Could you check a few things on this drawing? It's one solid part, dimensions in mm from its lowest x, y, z. Coordinates: 2 decimals unless noted, no trailing zeros. Loops run counter-clockwise (first coordinate to the right, second up) from the corner with the lowest first, then second, coordinate; pieces in that order, holes last. Notation, with made-up numbers: M 41.25,60.25 L 66.25,60.25 A21 cw 66.25,81.25 Z; hole C 76,86.25 d5. An arc over 180 degrees is marked long. Use one line per item in the form item = value. Start each with the question number.
(1) Please list where these lines run through material, in increasing order: L1, parallel to X at y = 51.64, z = 0.65; L2, parallel to Y at x = 1.75, z = 1.5; L3, parallel to Y at x = 10.25, z = 0.55.
(2) Imagine slicing it at B-B, the plane x = 8.5. Please give me the cut outline in (y, z) (3 decimals).
(3) Imagine slicing it at D-D, the plane x = 13.45. State how many separate pieces and enclosed holes the cut face has, and give its area (3 significant figures).
(4) Imagine slicing it at A-A, the plane y = 10. Please give me the cut outline in (x, z).
(5) Will these pins go through, and if not, where does the flat tip stop? P1, Ø1, axis at x = 7.5, z = 1, coming from the -Y side; P2, Ø0.6, axis at y = 77, z = 0.5, coming from the +X side; P3, Ø1, axis at y = 3.5, z = 1, coming from the -X side.
(6) Imagine slicing it at C-C, the plane y = 31.64. Please give me the cut outline in (x, z).
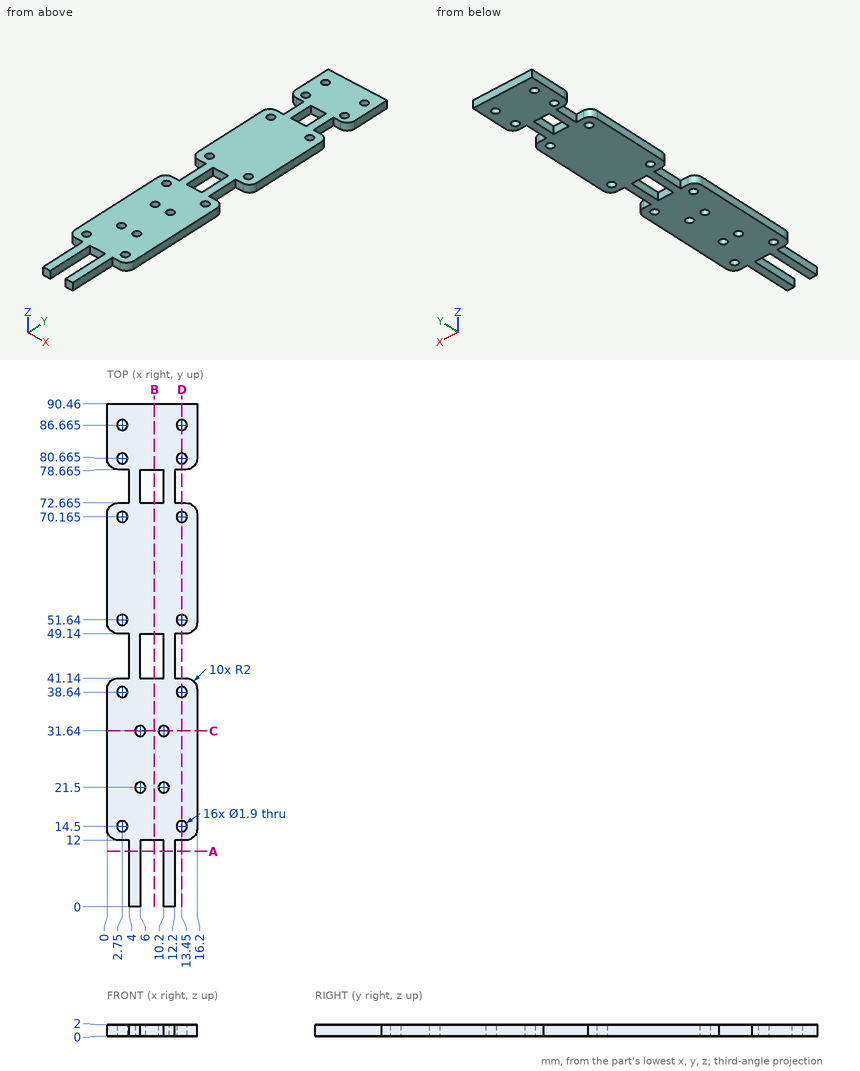
Answer:
q1.L1 = 0 to 1.8, 3.7 to 12.5, 14.4 to 16.2
q1.L2 = 12.02 to 41.12, 49.16 to 72.65, 78.68 to 90.46
q1.L3 = 0 to 20.55, 22.45 to 30.69, 32.59 to 90.46
q2.outline = M 12,0 L 41.14,0 L 41.14,2 L 12,2 Z; M 49.14,0 L 72.665,0 L 72.665,2 L 49.14,2 Z; M 78.665,0 L 90.46,0 L 90.46,2 L 78.665,2 Z
q3.separate_pieces = 9
q3.enclosed_holes = 0
q3.area = 106 mm²
q4.outline = M 4,0 L 6,0 L 6,2 L 4,2 Z; M 10.2,0 L 12.2,0 L 12.2,2 L 10.2,2 Z
q5.P1 = 12
q5.P2 = 12.2
q5.P3 = 4
q6.outline = M 0,0 L 5.05,0 L 5.05,2 L 0,2 Z; M 6.95,0 L 9.25,0 L 9.25,2 L 6.95,2 Z; M 11.15,0 L 16.2,0 L 16.2,2 L 11.15,2 Z
